Could you check a few things on this model? Use its own coordinates, in mm. A direction names the side the tool comes from. Coordinates: 2 decimals unless noted, no trailing zeros. Write each loop counter-clockwise with the first axis right and the second up, starting at its lowest first coordinate (ties: lowest second). Pieces come first, ordered by that corner, then holes.
Item 1: Thinking about a two-plate mould opening in Y: for faces 6 (the flat face through (-580, 30, -239)), 7 (the flat face through (-580, 0, 195)), 8 (the flat face through (-585, 0, -281.612)), which applies, +Y half, -Y half, draft (parallel to the pull), parting line (faces both ways), or undercut?
Item 2: If I drill on probe 1 along X at (y, z) = (20.5, -15); probe 2 along X at (y, z) = (16.5, 231); probe 3 along X at (y, z) = (2, -32), over which ranges is the centre line in solid material (lowest first)?
Item 3: I want a section at B-B on x = 50. Please give me the cut outline in (y, z).
Item 4: Which directions (+Z, -Z, +X, -X, +Y, -Y) give clear straight access to the entire face, cutting with the end or side of a thin tool? Please do faces 1 (the flat face through (-350, 0, -270)), 2 (the flat face through (28, -50, -1)), 3 (the flat face through (-580, 0, -195)), 4 (the flat face through (-585, 20, 241)), 5 (the flat face through (-580, 0, -285)).
Item 5: I want a section at D-D on z = 240. Please give me the cut outline in (x, y).
Item 6: For P1, Ø11, axis at y = -15.5, z = 237, coming from the +X side; P2, Ø3, axis at y = 0, z = -113, coming from the +X side; P3, Ø3, axis at y = -15, z = 234.5, coming from the -X side, each with a flat end and sliding along its axis, tell me the tip position at first contact or that it passes through.
Item 7: I want a section at A-A on z = 0. Please give me the cut outline in (x, y), then the cut area to 3 significant figures.
from build123d import *

# Parameters (mm, degrees)
SKETCH1_W           = 400
SKETCH1_H           = 25
SKETCH2_W           = 25
SKETCH2_H           = 540
SKETCH4_R           = 50
BOSS_EXTRUDE1_DEPTH = 50
SKETCH5_W           = 200
SKETCH5_H           = 10
SKETCH6_R           = 20
CUT_EXTRUDE1_DEPTH  = 621.805927955
SKETCH7_W           = 70
SKETCH7_H           = 90
BOSS_EXTRUDE2_DEPTH = 30
CUT_EXTRUDE2_DEPTH  = 20
SKETCH10_W          = 53.225586826
SKETCH10_H          = 20
CUT_EXTRUDE3_DEPTH  = 40


with BuildPart() as part:
    # Sketch1 → Revolve1 (revolve)
    with BuildSketch(Plane(origin=(0, 0, 0), x_dir=(1, 0, 0), z_dir=(0, 1, 0))):
        with Locations((-150, -12.5)):
            Rectangle(SKETCH1_W, SKETCH1_H)
    revolve(axis=Axis((-350, 0, 0), (1, 0, 0)))

    # Sketch2 → Revolve2 (revolve)
    with BuildSketch(Plane(origin=(0, 0, 0), x_dir=(1, 0, 0), z_dir=(0, 1, 0)), mode=Mode.PRIVATE) as revolve2_sk:
        with Locations((-362.5, 0)):
            Rectangle(SKETCH2_W, SKETCH2_H)
    revolve(revolve2_sk.sketch.rotate(Axis((-350, 0, 270), (0, 0, -1)), 180), axis=Axis((-350, 0, 270), (0, 0, -1)))

    # Sketch4 → Boss-Extrude1 (add, symmetric)
    with BuildSketch(Plane(origin=(0, 0, 0), x_dir=(1, 0, 0), z_dir=(0, 1, 0))):
        with Locations(Location((50, 0, 0), (0, 0, 270))):
            Circle(SKETCH4_R)
    extrude(amount=BOSS_EXTRUDE1_DEPTH, both=True)

    # Sketch5 → Revolve-Thin1 (revolve)
    with BuildSketch(Plane(origin=(0, 0, 0), x_dir=(1, 0, 0), z_dir=(0, 1, 0)), mode=Mode.PRIVATE) as revolve_thin1_sk:
        with Locations((-450, 235)):
            Rectangle(SKETCH5_W, SKETCH5_H)
    revolve_thin1 = revolve(revolve_thin1_sk.sketch.rotate(Axis((-350, 0, -240), (-1, 0, 0)), 180), axis=Axis((-350, 0, -240), (-1, 0, 0)))

    # Mirror2: Revolve-Thin1 across plane
    add(revolve_thin1.mirror(Plane.XY))

    # Sketch6 → Cut-Extrude1 (cut, through all)
    with BuildSketch(Plane(origin=(0, 50, 0), x_dir=(1, 0, 0), z_dir=(0, 1, 0))):
        with Locations(Location((50, 0, 0), (0, 0, 270))):
            Circle(SKETCH6_R)
    extrude(amount=-CUT_EXTRUDE1_DEPTH, mode=Mode.SUBTRACT)

    # Sketch7 → Boss-Extrude2 (add, symmetric)
    with BuildSketch(Plane(origin=(0, 0, 0), x_dir=(1, 0, 0), z_dir=(0, 1, 0))):
        with Locations((-580, -240)):
            Rectangle(SKETCH7_W, SKETCH7_H)
    boss_extrude2 = extrude(amount=BOSS_EXTRUDE2_DEPTH, both=True)

    # Sketch9 → Cut-Extrude2 (cut, symmetric)
    with BuildSketch(Plane(origin=(0, 0, 0), x_dir=(1, 0, 0), z_dir=(0, 1, 0))):
        Polygon((-575, -281.612233807), (-615, -281.612233807), (-615, -201.612233807), (-575, -201.612233807), (-555, -201.612233807), (-555, -281.612233807), align=None)
        with BuildLine():
            Line((-598, -265), (-602, -265))
            ThreePointArc((-602, -265), (-604.121320344, -264.121320344), (-605, -262))
            Line((-605, -262), (-605, -221.224467614))
            ThreePointArc((-605, -221.224467614), (-604.121320344, -219.103147271), (-602, -218.224467614))
            Line((-602, -218.224467614), (-598, -218.224467614))
            ThreePointArc((-598, -218.224467614), (-595.878679656, -219.103147271), (-595, -221.224467614))
            Line((-595, -221.224467614), (-595, -262))
            ThreePointArc((-595, -262), (-595.878679656, -264.121320344), (-598, -265))
        make_face(mode=Mode.SUBTRACT)
    cut_extrude2 = extrude(amount=CUT_EXTRUDE2_DEPTH, both=True, mode=Mode.SUBTRACT)

    # Sketch10 → Cut-Extrude3 (cut)
    with BuildSketch(Plane.ZY.offset(605)):
        with Locations((240, 0)):
            Rectangle(SKETCH10_W, SKETCH10_H)
    cut_extrude3 = extrude(amount=-CUT_EXTRUDE3_DEPTH, mode=Mode.SUBTRACT)

    # Mirror3: Boss-Extrude2, Cut-Extrude2, Cut-Extrude3 across plane
    add(boss_extrude2.mirror(Plane.XY))
    add(cut_extrude2.mirror(Plane.XY), mode=Mode.SUBTRACT)
    add(cut_extrude3.mirror(Plane.XY), mode=Mode.SUBTRACT)


solid = part.part
Response values:
1. face 6: +Y half
1. face 7: draft
1. face 8: undercut
2. probe 1: x = -364.31 to -335.69, 2.3 to 36.77, 63.23 to 97.7
2. probe 2: x = -605 to -595, -555 to -545, -368.78 to -331.22
2. probe 3: x = -374.92 to -325.08, 11.58 to 88.42
3. outline: (-50, -50) - (50, -50) - (50, -20) - (-50, -20) - close; (-50, 20) - (50, 20) - (50, 50) - (-50, 50) - close
4. face 1: -Z, +X, +Y, -Y
4. face 2: +Z, -Z, +X, -X, -Y
4. face 3: -X, +Y, -Y
4. face 4: none
4. face 5: -Z, +X, -X, +Y, -Y
5. outline: (-615, -30) - (-545, -30) - (-545, -10) - (-372.91, -10) arc R25 ccw (long way) to (-372.91, 10) - (-545, 10) - (-545, 30) - (-615, 30) - (-615, 20) - (-605, 20) - (-605, 10) - (-595, 10) - (-595, 20) - (-555, 20) - (-555, -20) - (-595, -20) - (-595, -10) - (-605, -10) - (-605, -20) - (-615, -20) - close
6. P1: stops at x = -327.09
6. P2: stops at x = -325
6. P3: stops at x = -605
7. outline: (-350, -25) - (0, -25) - (0, -50) - (30, -50) - (30, 50) - (0, 50) - (0, 25) - (-350, 25) arc R25 ccw to start; (70, -50) - (100, -50) - (100, 50) - (70, 50) - close
7. area: 24,500 mm2
